Design review of the part shown in the three views and the two pictorial views. Dimensions are in mm from the part's minimum x, y and z. A direction names the side the tool comes from. Round coordinates to 2 decimals unless told otherwise and drop trailing zeros. Loops run counter-clockwise (first coordinate to the right, second up) from the corner with the lowest first, then second, coordinate; pieces in that order, holes last. Notation, with made-up numbers: (52, -28.5) -> (90, -28.5) arc R15 ccw to (90, -13.5) -> close; hole circle Ø6 at (58.25, -14). An arc over 180 degrees is marked (long way). Use a Markdown table: item, result. Add a question column.
1) Insertion check: pin 1 (1.5 mm diameter, centred on y = 8.5, z = 2, fed in from -X); pin 2 (8 mm diameter, centred on y = 13.5, z = 1.5, fed in from +X); pin 3 (5 mm diameter, centred on x = 13, y = 7.5, fed in from +Z). Each pin has a flat end and moves straight along its axis. Give the tip position at first contact, or say it passes through.
2) Consider section C-C on y = 12.5. Give the boundary of the cut face in (x, z), plus the area to 3 significant figures.
3) Consider section B-B on x = 22. Give the boundary of the cut face in (y, z), plus the area to 3 significant figures.
4) Wall thickness on probe 1 along Y at (x, z) = (13, 8.5); probe 2 along X at (y, z) = (9.5, 3.75); probe 3 along X at (y, z) = (1.5, 10): over which ranges is each line inside the solid? List them lowest first.
5) Consider section D-D on z = 2.5. Give the boundary of the cut face in (x, y).
6) For the marked faces 4, 5 and 6, list the 3-axis set-ups (+Z, -Z, +X, -X, +Y, -Y) from which the entire face can be reached by the end or side of a thin tool; tool diameter is ignored.
7) Mouldability with a two-part tool opening along Y and no side actions: class the marked faces 1, 2 and 3 as released by +Y, released by -Y, zero draft, split by the parting line, or undercut.
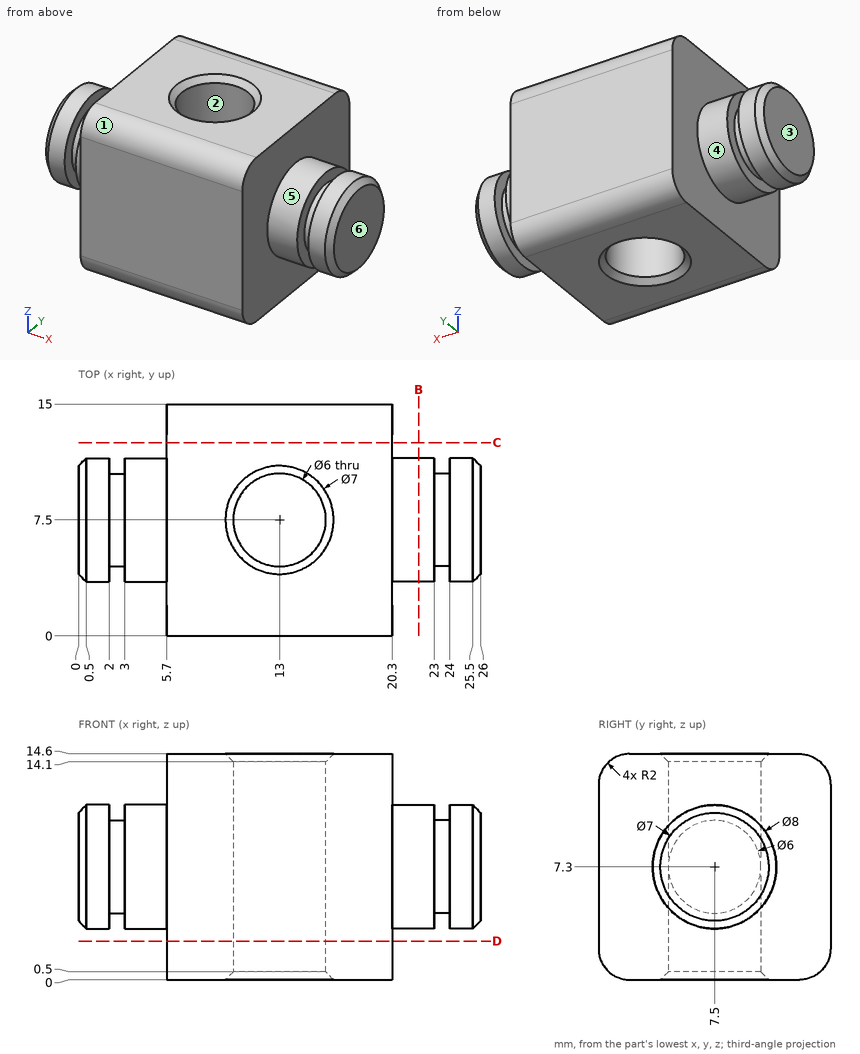
Result set:
| question | item | result |
|---|---|---|
| 1 | pin 1 | x = 5.7 |
| 1 | pin 2 | x = 20.3 |
| 1 | pin 3 | through |
| 2 | outline | (5.7, 0) -> (20.3, 0) -> (20.3, 14.6) -> (5.7, 14.6) -> close |
| 2 | area | 213 mm2 |
| 3 | outline | circle Ø8 at (7.5, 7.3) |
| 3 | area | 50.3 mm2 |
| 4 | probe 1 | 0 to 4.5, 10.5 to 15 |
| 4 | probe 2 | 5.7 to 10.76, 15.24 to 20.3 |
| 4 | probe 3 | 5.7 to 20.3 |
| 5 | outline | (5.7, 0) -> (20.3, 0) -> (20.3, 15) -> (5.7, 15) -> close; hole circle Ø6 at (13, 7.5) |
| 6 | face 4 | -X |
| 6 | face 5 | +X |
| 6 | face 6 | +Z, -Z, +X, +Y, -Y |
| 7 | face 1 | released by -Y |
| 7 | face 2 | undercut |
| 7 | face 3 | zero draft |
